from build123d import *

# Parameters (mm, degrees)
F1_R     = 50
F1_R_2   = 25
F2_DEPTH = 18
F4_R     = 50
F4_R_2   = 25
F4_R_3   = 15
F5_DEPTH = 18


with BuildPart() as f2:
    # F1 (on Right) → F2 (new body)
    with BuildSketch(Plane.YZ):
        with Locations((0, -59.5)):
            Circle(F1_R)
        with Locations((0, -59.5)):
            Circle(F1_R_2, mode=Mode.SUBTRACT)
        with Locations((0, -59.5)):
            Circle(F1_R_2)
        with BuildLine():
            ThreePointArc((0, -44.5), (10.6066017178, -48.8933982822), (15, -59.5))
            ThreePointArc((15, -59.5), (-10.6066017178, -70.1066017178), (0, -44.5))
        make_face(mode=Mode.SUBTRACT)
    extrude(amount=-F2_DEPTH)

    # F3: sweep along a path in F0
    with BuildLine(Plane.XZ) as f3_path:
        ThreePointArc((0, -59.5), (22.7696642257, -54.9708321844), (42.0728534806, -42.0728534806))
    # F1 (on Right) → F3 (sweep)
    with BuildSketch(Plane.YZ):
        with Locations((0, -59.5)):
            Circle(F1_R_2)
        with BuildLine():
            ThreePointArc((0, -44.5), (10.6066017178, -48.8933982822), (15, -59.5))
            ThreePointArc((15, -59.5), (-10.6066017178, -70.1066017178), (0, -44.5))
        make_face(mode=Mode.SUBTRACT)
    sweep(path=f3_path.line)

    # F4 (on face) → F5 (join)
    with BuildSketch(Plane(origin=(0, 0, 0), x_dir=(0, 1, 0), z_dir=(0.7071067812, 0, 0.7071067812))):
        with Locations((0, -59.5)):
            Circle(F4_R)
        with Locations((0, -59.5)):
            Circle(F4_R_2, mode=Mode.SUBTRACT)
        with Locations((0, -59.5)):
            Circle(F4_R_2)
        with Locations((0, -59.5)):
            Circle(F4_R_3, mode=Mode.SUBTRACT)
    extrude(amount=F5_DEPTH)


solid = f2.part
Can you work these out from the model? Positions are in its coordinate system, mm. A direction names the side the tool comes from. Coordinates: 2 decimals unless noted, no trailing zeros. Write each loop counter-clockwise with the first axis right and the second up, starting at its lowest first coordinate (ties: lowest second). Pieces come first, ordered by that corner, then holes. Notation, with made-up numbers: (-37, 33) -> (17, 33) arc R8 ccw to (17, 39) -> close; hole circle Ø10 at (63, -38.5). An arc over 180 degrees is marked (long way). Answer as CSV lines item,"result".
1) Will these pins go through, and if not, where does the flat tip stop? P1, Ø1, axis at y = 39, z = -17, coming from the +X side; P2, Ø6, axis at y = -27.5, z = -95.5, coming from the +X side; P3, Ø3, axis at x = 27.5, y = -36.5, coming from the -Z side.
Check result:
P1,"x = 42.96"
P2,"x = 0"
P3,"z = -29"
2) If we mould it in two halves opening along X, with no side actions, what happens to faces 3 (the cylindrical face through (58.702, -3.252, -46.152)), 4 (the flat face through (-18, -12, -70)), 5 (the cylindrical face through (-8.874, -3.252, -44.857)), 6 (the flat face through (46.449, 10.411, -20.993))? For each: +X half, -X half, draft (parallel to the pull), parting line (faces both ways), or undercut.
Check result:
face 3,"undercut"
face 4,"-X half"
face 5,"draft"
face 6,"+X half"
3) If we section it at A-A on y = 13.5: Please give me the cut outline in (x, z), then the cut area to 3 significant figures.
Check result:
outline,"(-18, -107.64) -> (0, -107.64) -> (0, -80.54) arc R80.54 ccw to (56.95, -56.95) -> (76.12, -76.12) -> (88.84, -63.39) -> (59.42, -33.97) -> (46.7, -46.7) arc R66.04 cw to (0, -66.04) -> (-18, -66.04) -> close; (-18, -52.96) -> (0, -52.96) arc R52.96 ccw to (37.45, -37.45) -> (50.18, -24.72) -> (20.76, 4.7) -> (8.03, -8.03) -> (27.19, -27.19) arc R38.46 cw to (0, -38.46) -> (0, -11.36) -> (-18, -11.36) -> close"
area,"4,350 mm²"
4) If I drill on line 1 (Z direction, x = -5, y = 0); line 2 (Y direction, x = -5, z = -59); line 3 (X direction, y = 12, z = -21.5), over which ranges is the centre line in solid material (lowest first)? Write a range as from..to.
Check result:
line 1,"-109.5..-74.5, -44.5..-9.5"
line 2,"-50..-14.99, 14.99..50"
line 3,"-18..0, 21.5..46.96"
5) If we section it at C-C on x = 15.5: Count the separate pieces of the cut face and the enclosed holes in it, then the cut area to 3 significant figures.
Check result:
separate pieces,"2"
enclosed holes,"1"
area,"2,110 mm²"
6) If we section it at B-B on y = 0: Please give me the cut outline in (x, z), then the cut area to 3 significant figures.
Check result:
outline,"(-18, -109.5) -> (0, -109.5) -> (0, -84.5) arc R84.5 ccw to (59.75, -59.75) -> (77.43, -77.43) -> (90.16, -64.7) -> (65.41, -39.95) -> (52.68, -52.68) arc R74.5 cw to (0, -74.5) -> (-18, -74.5) -> close; (-18, -44.5) -> (0, -44.5) arc R44.5 ccw to (31.47, -31.47) -> (44.19, -18.74) -> (19.45, 6.01) -> (6.72, -6.72) -> (24.4, -24.4) arc R34.5 cw to (0, -34.5) -> (0, -9.5) -> (-18, -9.5) -> close"
area,"3,450 mm²"
7) On a 3-axis mill with a long thin cutter (end or side, diameter ignored), from which of +Z, -Z, +X, -X, +Y, -Y can I reach the whole of each face in a straight line? I mean faces 1 (the cylindrical face through (-8.87, -10.84, -108.31)), 2 (the flat face through (0, -23, -70)). Say none if no direction works.
Check result:
face 1,"-X"
face 2,"none"
8) If we section it at D-D on y = -20.5: Please give me the cut outline in (x, z).
Check result:
outline,"(-18, -105.1) -> (0, -105.1) -> (0, -73.81) arc R73.81 ccw to (52.19, -52.19) -> (74.32, -74.32) -> (87.05, -61.59) -> (22.55, 2.9) -> (9.83, -9.83) -> (31.95, -31.95) arc R45.19 cw to (0, -45.19) -> (0, -13.9) -> (-18, -13.9) -> close"
